Can you work these out from the model? Positions are in its coordinate system, mm. A direction names the side the tool comes from. Give positions to 0.01 mm unless a question says otherwise; leave off trailing zeros. Loops run counter-clockwise (first coordinate to the right, second up) from the corner with the lowest first, then second, coordinate; pieces in that order, holes last. Notation, with made-up numbers: M -20,64.25 L 7,64.25 A29 cw 7,90.25 Z; hole C 81.5,-8.5 d8. An arc over 180 degrees is marked long. Answer as a JSON object with one key per item and string values.
```python
from build123d import *

# Parameters (mm, degrees)
SKETCH1_R           = 1
SKETCH1_W           = 39.213246084
SKETCH1_H           = 2
SKETCH1_W_2         = 45.726803631
SKETCH1_W_3         = 2
SKETCH1_H_2         = 19.484553002
BOSS_EXTRUDE1_DEPTH = 2
FILLET1_R           = 3


with BuildPart() as part:
    # Sketch1 → Boss-Extrude1 (new body)
    with BuildSketch(Plane(origin=(0, 0, 0), x_dir=(1, 0, 0), z_dir=(0, 1, 0))):
        Polygon((-5, 3), (-5, 12), (5, 12), (5, 3), (60, 3), (60, -3), (5, -3), (5, -12), (-5, -12), (-5, -3), (-60, -3), (-60, 3), align=None)
        with Locations(Location((-57, 0.057494984, 0), (0, 0, 270))):
            Circle(SKETCH1_R, mode=Mode.SUBTRACT)
        with Locations((-31.867954369, 0.057494984)):
            Rectangle(SKETCH1_W, SKETCH1_H, mode=Mode.SUBTRACT)
        with Locations((32.832738322, 0.057494984)):
            Rectangle(SKETCH1_W_2, SKETCH1_H, mode=Mode.SUBTRACT)
        Rectangle(SKETCH1_W_3, SKETCH1_H_2, mode=Mode.SUBTRACT)
    extrude(amount=BOSS_EXTRUDE1_DEPTH)

    # Fillet1
    fillet1_edges = [part.edges().sort_by_distance(p)[0] for p in [
        (-60, 1, 3),
        (-60, 1, -3),
    ]]
    fillet(fillet1_edges, radius=FILLET1_R - 0.0001)  # a hair under: the kernel refuses the full size


solid = part.part
```
1) Suppose I cut it at B-B, the plane y = 0.7. Give the number of separate pieces and of enclosed holes in the cut face, and give its area (3 significant figures).
Answer list:
{"separate pieces": "1", "enclosed holes": "4", "area": "684 mm^2"}
2) Suppose I cut it at D-D, the plane x = -9.5. Write out the boundary of the cut face in (y, z).
Answer list:
{"outline": "M 0,-3 L 2,-3 L 2,3 L 0,3 Z"}
3) Please list where these lines run through material, in increasing order: line 1 along X through (y, z) = (0.4, -6); line 2 along Z through (x, y) = (-40, 1.8); line 3 along X through (y, z) = (1.7, 1.75). Write a range as from..to.
Answer list:
{"line 1": "-5..-1, 1..5", "line 2": "-3..-1.06, 0.94..3", "line 3": "-59.44..-1, 1..60"}
4) For faces 5 (the cylindrical face through (-59.1, 1.01, -2.14)), 6 (the flat face through (32, 1, -3)), 7 (the flat face through (-31, 1, 3)), 8 (the flat face through (9.969, 1, 0)), 9 (the flat face through (33, 1, 3)), which set-ups out of +Z, -Z, +X, -X, +Y, -Y let a thin tool reach every point of the face, with its end or its side?
Answer list:
{"face 5": "-Z, -X, +Y, -Y", "face 6": "-Z, +X, +Y, -Y", "face 7": "+Z, -X, +Y, -Y", "face 8": "+Y, -Y", "face 9": "+Z, +X, +Y, -Y"}
5) Will these pins go through, and if not, where does the flat tip stop? pin 1 Ø1 at (x, y) = (31, 0.5) entering from +Z; pin 2 Ø0.6 at (x, y) = (26.5, 1.5) entering from -Z; pin 3 Ø1 at (y, z) = (1, -6.5) entering from +X.
Answer list:
{"pin 1": "z = 3", "pin 2": "z = -3", "pin 3": "x = 5"}
6) Suppose I cut it at A-A, the plane x = -43. Write out the boundary of the cut face in (y, z), and give its area (3 significant figures).
Answer list:
{"outline": "M 0,-3 L 2,-3 L 2,-1.06 L 0,-1.06 Z; M 0,0.94 L 2,0.94 L 2,3 L 0,3 Z", "area": "8.00 mm^2"}
7) If we mould it in two halves opening along X, with no side actions, what happens to faces 1 (the flat face through (55.696, 1, 0)), 2 (the flat face through (-4, 0, 1)), 3 (the flat face through (0, 1, 9.742)), 4 (the cylindrical face through (-59.14, 1.01, 2.1))? For each: +X half, -X half, draft (parallel to the pull), parting line (faces both ways), or undercut.
Answer list:
{"face 1": "undercut", "face 2": "draft", "face 3": "undercut", "face 4": "-X half"}
8) Suppose I cut it at C-C, the plane z = -7.5. Write out the boundary of the cut face in (x, y), and give its area (3 significant figures).
Answer list:
{"outline": "M -5,0 L -1,0 L -1,2 L -5,2 Z; M 1,0 L 5,0 L 5,2 L 1,2 Z", "area": "16.0 mm^2"}
